```python
from build123d import *

# Parameters (mm, degrees)
ESQUISSE1_W             = 100
ESQUISSE1_H             = 41
BOSS_EXTRU_1_DEPTH      = 3
ESQUISSE2_W             = 7
ESQUISSE2_H             = 11
ENL_V_MAT_EXTRU_2_DEPTH = 3
ESQUISSE3_W             = 3
ESQUISSE3_H             = 15
BOSS_EXTRU_2_DEPTH      = 18
ESQUISSE4_R             = 7.5
ENL_V_MAT_EXTRU_3_DEPTH = 6


with BuildPart() as part:
    # Esquisse1 → Boss.-Extru.1 (new body)
    with BuildSketch(Plane(origin=(0, 0, 0), x_dir=(1, 0, 0), z_dir=(0, 1, 0))):
        Rectangle(ESQUISSE1_W, ESQUISSE1_H)
    extrude(amount=BOSS_EXTRU_1_DEPTH)

    # Esquisse2 → Enlèv. mat.-Extru.2 (cut)
    with BuildSketch(Plane(origin=(0, 3, 0), x_dir=(1, 0, 0), z_dir=(0, 1, 0))):
        with Locations((-36.5, 0)):
            Rectangle(ESQUISSE2_W, ESQUISSE2_H)
    extrude(amount=-ENL_V_MAT_EXTRU_2_DEPTH, mode=Mode.SUBTRACT)

    # Esquisse3 → Boss.-Extru.2 (add)
    with BuildSketch(Plane.XZ):
        with Locations((48.5, -9.5)):
            Rectangle(ESQUISSE3_W, ESQUISSE3_H)
    extrude(amount=-BOSS_EXTRU_2_DEPTH)

    # Esquisse4 → Enlèv. mat.-Extru.3 (cut)
    with BuildSketch(Plane(origin=(50, 0, 0), x_dir=(0, 0, -1), z_dir=(1, 0, 0))):
        with Locations((9.5, 18)):
            Circle(ESQUISSE4_R)
    extrude(amount=-ENL_V_MAT_EXTRU_3_DEPTH, mode=Mode.SUBTRACT)


solid = part.part
```
Geometry: final body of the model. Coordinates: model frame, mm. A direction names the side the tool comes from. Give positions to 0.01 mm unless a question says otherwise; leave off trailing zeros. Write each loop counter-clockwise with the first axis right and the second up, starting at its lowest first coordinate (ties: lowest second). Pieces come first, ordered by that corner, then holes.
1. Section query C-C, the plane z = -9.5. Return loops of the section in (x, y).
2. Pin query (flat end, axial travel): P1, Ø5, axis at x = -17, z = -12.5, coming from the +Y side; P2, Ø2.5, axis at x = 48, y = 10.5, coming from the -Z side; P3, Ø8, axis at y = 8, z = -10.5, coming from the -X side; P4, Ø4, axis at y = 4, z = 5, coming from the -X side. Return the tip coordinate at first contact, or that it passes through.
3. Section query B-B, the plane z = 2.5. Return loops of the section in (x, y).
4. Reachability of faces 4 (the flat face through (-40, 2, 0)), 5 (the flat face through (48, 10, -17)), 6 (the flat face through (48, 10, -2)) from +Z, -Z, +X, -X, +Y, -Y: full face, straight path, thin tool, end or side. Return the list, or none.
5. Section query D-D, the plane y = 8.25. Return loops of the section in (x, z).
6. Line query: probe 1 along X at (y, z) = (2.5, 1); probe 2 along Y at (x, z) = (-28.5, 3.5). Output: solid intervals per line, ascending.
7. Section query A-A, the plane x = -34.5. Return loops of the section in (y, z).
8. Draft query along Z for faces 1 (the flat face through (-33, 2, 0)), 2 (the flat face through (-1, 1, 20.5)), 3 (the flat face through (47, 7, -10)). Return one class per face: released by +Z, released by -Z, zero draft, split by the parting line, or undercut.
Computed:
1. outline: (-50, 0) - (50, 0) - (50, 10.5) - (47, 10.5) - (47, 3) - (-50, 3) - close
2. P1: stops at y = 3
2. P2: stops at z = -17
2. P3: stops at x = 47
2. P4: stops at x = -50
3. outline: (-50, 0) - (-40, 0) - (-40, 3) - (-50, 3) - close; (-33, 0) - (50, 0) - (50, 3) - (-33, 3) - close
4. face 4: +Y, -Y
4. face 5: -Z, +X, -X, +Y
4. face 6: +Z, +X, -X, +Y
5. outline: (47, -17) - (50, -17) - (50, -2) - (47, -2) - close
6. probe 1: x = -50 to -40, -33 to 50
6. probe 2: y = 0 to 3
7. outline: (0, -20.5) - (3, -20.5) - (3, -5.5) - (0, -5.5) - close; (0, 5.5) - (3, 5.5) - (3, 20.5) - (0, 20.5) - close
8. face 1: undercut
8. face 2: released by +Z
8. face 3: zero draft
